Autodesk Inventor part; units mm, degrees
ref_plane "YZ Plane" through (0, 0, 0) normal (1, 0, 0) x (0, 1, 0)
ref_plane "XZ Plane" through (0, 0, 0) normal (0, 1, 0) x (-1, 0, 0)
ref_plane "XY Plane" through (0, 0, 0) normal (0, 0, 1) x (1, 0, 0)
sketch "Sketch1" plane through (0, 0, 0) normal (0, 0, 1) x (1, 0, 0)
  line L0 (-165.1, 298.45) -> (165.1, 298.45)
  line L1 (165.1, 298.45) -> (165.1, -298.45)
  line L2 (165.1, -298.45) -> (-165.1, -298.45)
  line L3 (-165.1, -298.45) -> (-165.1, 298.45)
  point P0 (0, 0)
  point P1 (0, 298.45)
  point P2 (-165.1, 0)
  dimension "d0" = 330.2
  dimension "d1" = 596.9
extrude "Extrusion1" add sketch "Sketch1" along normal blind 3
sketch "Sketch2" plane through (0, 0, 3) normal (0, 0, 1) x (1, 0, 0)
  line L0 (165.1, 298.45) -> (165.1, -298.45)
  line L1 (-165.1, 298.45) -> (165.1, 298.45)
  line L2 (-165.1, -298.45) -> (-165.1, 298.45)
  line L3 (165.1, -298.45) -> (-165.1, -298.45)
  line L4 (-139.7, 273.05) -> (139.7, 273.05)
  line L5 (139.7, 273.05) -> (139.7, -273.05)
  line L6 (139.7, -273.05) -> (-139.7, -273.05)
  line L7 (-139.7, -273.05) -> (-139.7, 273.05)
  point P0 (0, 0)
  dimension "d4" = 25.4
  dimension "d5" = 25.4
  dimension "d6" = 25.4
  dimension "d7" = 25.4
extrude "Extrusion2" cut sketch "Sketch2" against normal blind 3 contours L4 L5 L6 L7
properties part number "inside lining"
Verification items for the finished model (mm, model axes). Round coordinates to 2 decimals unless told otherwise and drop trailing zeros. Loops run counter-clockwise (first coordinate to the right, second up) from the corner with the lowest first, then second, coordinate; pieces in that order, holes last. Notation, with made-up numbers: (57.25, -5) - (78.25, -5) arc R20 ccw to (78.25, 27) - close; hole circle Ø3 at (-29, 11). An arc over 180 degrees is marked (long way). Answer in a Markdown table with one row per item. Add a question column.
Q1. Section check B-B on z = 1.3. Enter the section's corners in (x, y).
Q2. Section check A-A on x = 77.5. Enter the section's corners in (y, z), plus the area to 3 significant figures.
Q3. Section check C-C on y = -123.5. Enter the section's corners in (x, z).
Q4. Material ranges on line 1 (Y direction, x = 67, z = 0.9); line 2 (X direction, y = -224, z = 1.2), recorded low to high.
Found:
| question | item | result |
|---|---|---|
| 1 | outline | (-165.1, -298.45) - (165.1, -298.45) - (165.1, 298.45) - (-165.1, 298.45) - close; hole (-139.7, -273.05) - (139.7, -273.05) - (139.7, 273.05) - (-139.7, 273.05) - close |
| 2 | outline | (-298.45, 0) - (-273.05, 0) - (-273.05, 3) - (-298.45, 3) - close; (273.05, 0) - (298.45, 0) - (298.45, 3) - (273.05, 3) - close |
| 2 | area | 152 mm² |
| 3 | outline | (-165.1, 0) - (-139.7, 0) - (-139.7, 3) - (-165.1, 3) - close; (139.7, 0) - (165.1, 0) - (165.1, 3) - (139.7, 3) - close |
| 4 | line 1 | y = -298.45 to -273.05, 273.05 to 298.45 |
| 4 | line 2 | x = -165.1 to -139.7, 139.7 to 165.1 |
